Input: part model. Units: mm. Frame: model coordinates. A direction names the side the tool comes from. Give positions to 0.01 mm unless a question says otherwise; leave off trailing zeros. Order: outer loops, then holes, each group sorted by start corner. A loop starts at its lowest first (then second) coordinate and runs counter-clockwise, first axis right, second up.
```python
from build123d import *


with BuildPart() as part:
    # Sketch1 → Revolve1 (revolve)
    with BuildSketch(Plane.XY):
        with BuildLine():
            Line((0, 0), (0, 8.58901))
            Line((0, 8.58901), (0.93599, 9.525))
            Line((0.93599, 9.525), (9.310047461, 9.525))
            Line((9.310047461, 9.525), (10.262333187, 8.610821042))
            ThreePointArc((10.262333187, 8.610821042), (10.619173954, 8.380210754), (11.0363, 8.29945))
            Line((11.0363, 8.29945), (12.3698, 8.29945))
            ThreePointArc((12.3698, 8.29945), (13.160062539, 8.626787461), (13.4874, 9.41705))
            Line((13.4874, 9.41705), (13.4874, 9.49325))
            Line((13.4874, 9.49325), (15.875, 9.49325))
            Line((15.875, 9.49325), (15.875, 0))
            Line((15.875, 0), (0, 0))
        make_face()
    revolve(axis=Axis((15.875, 0, 0), (-1, 0, 0)))

    # Sketch2 → Revolve2 (revolve)
    with BuildSketch(Plane.XY):
        Polygon((15.875, 0), (15.875, 19.00555), (16.637, 19.76755), (41.2115, 19.76755), (41.2115, 18.18005), (42.2275, 18.18005), (43.2435, 19.19605), (46.863, 19.19605), (47.625, 18.43405), (47.625, 0), align=None)
    revolve(axis=Axis((47.625, 0, 0), (-1, 0, 0)))

    # Sketch3 → Cut-Revolve1 (revolve, cut)
    with BuildSketch(Plane.XY):
        Polygon((0, 0), (0, 6.3754), (0.762, 5.6134), (47.625, 5.6134), (47.625, 0), align=None)
    revolve(axis=Axis((47.625, 0, 0), (-1, 0, 0)), mode=Mode.SUBTRACT)

    # Sketch4 → Cut-Revolve2 (revolve, cut)
    with BuildSketch(Plane(origin=(0, 0, 0), x_dir=(1, 0, 0), z_dir=(0, 1, 0))):
        Polygon((31.75, 0), (34.925, 0), (34.925, -7.768124148), (36.256425852, -9.09955), (36.589475925, -19.76755), (31.75, -19.76755), align=None)
    revolve(axis=Axis((31.75, 0, 19.76755), (0, 0, -1)), mode=Mode.SUBTRACT)

    # Sketch5 → Revolve3 (revolve)
    with BuildSketch(Plane.XY):
        with BuildLine():
            Line((41.2115, 18.888259175), (41.2115, 17.92605))
            Line((41.2115, 17.92605), (42.2275, 17.92605))
            Line((42.2275, 17.92605), (42.2275, 18.18005))
            Line((42.2275, 18.18005), (41.7195, 18.18005))
            Line((41.7195, 18.18005), (41.344882072, 18.554667928))
            ThreePointArc((41.344882072, 18.554667928), (41.307684633, 18.64447049), (41.344882072, 18.734273051))
            Line((41.344882072, 18.734273051), (42.293990825, 19.683381804))
            Line((42.293990825, 19.683381804), (42.293990825, 19.76755))
            Line((42.293990825, 19.76755), (42.090790825, 19.76755))
            Line((42.090790825, 19.76755), (41.2115, 18.888259175))
        make_face()
    revolve(axis=Axis((42.2275, 0, 0), (-1, 0, 0)))


solid = part.part
```
1) Pull-direction query (X, two-part tool) for faces 1 (the face through (47.625, 3.8, -4.4)), 2 (the face through (41.98, -3.94, 17.75)), 3 (the face through (5.182, -7.559, 5.796)); classes: pulls with the +X half, pulls with the -X half, needs draft (parallel to the pull), parting line crosses it, or undercut.
2) Line query: probe 1 along Z at (x, y) = (41.5, 16); probe 2 along Z at (x, y) = (37, 0). Output: solid intervals per line, ascending.
3) Cut plane D-D (x = 6). Return the cut outline in (y, z) (3 decimals).
4) Cut plane A-A (x = 24.5). Return the cut outline in (y, z).
5) Cut plane C-C (y = 0). Count the separate pieces of the cut face and the enclosed holes in it, then the cut area to 3 significant figures.
6) Cut plane B-B (x = 31.75). Return the cut outline in (y, z) (3 decimals).
7) Reachability of faces 4 (the face through (0, 1.3, -6.4)), 5 (the face through (36.21, -1.4, 14.51)) from +Z, -Z, +X, -X, +Y, -Y: full face, straight path, thin tool, end or side. Return the list, or none.
8) First-contact query: P1, Ø1, axis at y = -9.5, z = 15, coming from the -X side (3 decimals); P2, Ø10, axis at x = 20, z = 9, coming from the +Y side; P3, Ø12, axis at x = 11.5, y = -2, coming from the +Z side. Flat tips, straight axial feed; report the tip coordinate or a pass-through.
Geometry says:
1. face 1: pulls with the +X half
1. face 2: undercut
1. face 3: needs draft
2. probe 1: z = -10.57 to -10.04, -9.09 to 9.09, 10.04 to 10.57
2. probe 2: z = -19.77 to -5.61, 5.61 to 19.77
3. outline: circle Ø19.05 at (0, 0); hole circle Ø11.227 at (0, 0)
4. outline: circle Ø39.54 at (0, 0); hole circle Ø11.23 at (0, 0)
5. separate pieces: 3
5. enclosed holes: 0
5. area: 879 mm2
6. outline: (-4.821, 19.171) arc R19.768 ccw (long way) to (4.821, 19.171) - (4.506, 9.1) - (3.175, 7.768) - (3.175, 4.629) arc R5.613 cw (long way) to (-3.175, 4.629) - (-3.175, 7.768) - (-4.506, 9.1) - close
7. face 4: +Z, -Z, -X, +Y, -Y
7. face 5: +Z
8. P1: stops at x = 15.875
8. P2: stops at y = 19.36
8. P3: stops at z = 19.77
